Verification items for this drawing (mm, ordinates from the low corner). A direction names the side the tool comes from. Give positions to 0.01 mm unless a question says otherwise; leave off trailing zeros. Write each loop counter-clockwise with the first axis right and the second up, starting at its lowest first coordinate (ties: lowest second). Pieces come first, ordered by that corner, then holes. Notation, with made-up numbers: (29, 89) -> (82, 89) arc R20 cw to (82, 110) -> close; hole circle Ø2 at (78, -3.75). An arc over 180 degrees is marked (long way). Answer as a JSON object with one key per item and string values.
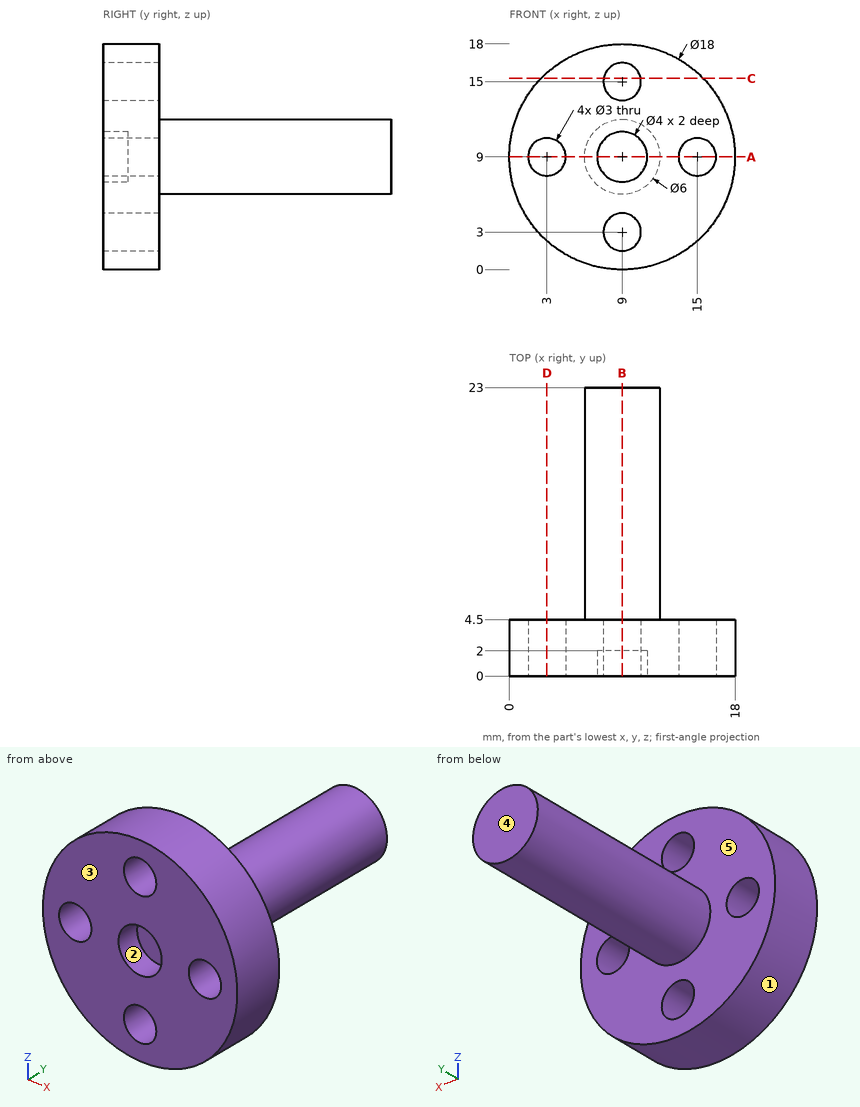
1. Sectioned sample at C-C, the plane z = 15.25. Enter the section's corners in (x, y), plus the area to 3 significant figures.
Determined:
{"outline": "(2.52, 0) -> (7.52, 0) -> (7.52, 4.5) -> (2.52, 4.5) -> close; (10.48, 0) -> (15.48, 0) -> (15.48, 4.5) -> (10.48, 4.5) -> close", "area": "45.0 mm^2"}
2. Access from +Z, -Z, +X, -X, +Y, -Y to the whole of each face (thin tool, end or side, straight path). Record for the marked faces 4 and 5.
Determined:
{"face 4": "+Z, -Z, +X, -X, +Y", "face 5": "+Y"}
3. Mould release check, pull along X, two halves, no side actions. Record for the marked faces 1, 2 and 3: released by +X, released by -X, zero draft, split by the parting line, or undercut.
Determined:
{"face 1": "split by the parting line", "face 2": "undercut", "face 3": "zero draft"}
4. Sectioned sample at B-B, the plane x = 9. Enter the section's corners in (y, z).
Determined:
{"outline": "(0, 0) -> (4.5, 0) -> (4.5, 1.5) -> (0, 1.5) -> close; (0, 4.5) -> (4.5, 4.5) -> (4.5, 6) -> (23, 6) -> (23, 12) -> (4.5, 12) -> (4.5, 13.5) -> (0, 13.5) -> (0, 11) -> (2, 11) -> (2, 7) -> (0, 7) -> close; (0, 16.5) -> (4.5, 16.5) -> (4.5, 18) -> (0, 18) -> close"}
5. Sectioned sample at D-D, the plane x = 3. Enter the section's corners in (y, z), plus the area to 3 significant figures.
Determined:
{"outline": "(0, 2.29) -> (4.5, 2.29) -> (4.5, 7.5) -> (0, 7.5) -> close; (0, 10.5) -> (4.5, 10.5) -> (4.5, 15.71) -> (0, 15.71) -> close", "area": "46.9 mm^2"}
6. Sectioned sample at A-A, the plane z = 9. Enter the section's corners in (x, y), plus the area to 3 significant figures.
Determined:
{"outline": "(0, 0) -> (1.5, 0) -> (1.5, 4.5) -> (0, 4.5) -> close; (4.5, 0) -> (7, 0) -> (7, 2) -> (11, 2) -> (11, 0) -> (13.5, 0) -> (13.5, 4.5) -> (12, 4.5) -> (12, 23) -> (6, 23) -> (6, 4.5) -> (4.5, 4.5) -> close; (16.5, 0) -> (18, 0) -> (18, 4.5) -> (16.5, 4.5) -> close", "area": "157 mm^2"}
7. Scan lines: L1, parallel to X at y = 1.55, z = 9; L2, parallel to X at y = 2.25, z = 10.25; L3, parallel to Y at x = 15, z = 4. Record each from-to range of solid material in increasing order. Write a range as [from, to].
Determined:
{"L1": "[0, 1.5], [4.5, 7], [11, 13.5], [16.5, 18]", "L2": "[0.09, 2.17], [3.83, 14.17], [15.83, 17.91]", "L3": "[0, 4.5]"}
8. Go/stop test with flat-tipped pins: P1, Ø3.5, axis at x = 9, z = 15, coming from the +Y side; P2, Ø1.8, axis at x = 15, z = 9, coming from the -Y side; P3, Ø2, axis at x = 12.5, y = 20.5, coming from the -Z side; P4, Ø6, axis at x = 8.5, y = 12, coming from the -Z side. Record where each tip stops, or that it passes through.
Determined:
{"P1": "y = 4.5", "P2": "through", "P3": "z = 7.34", "P4": "z = 6"}
